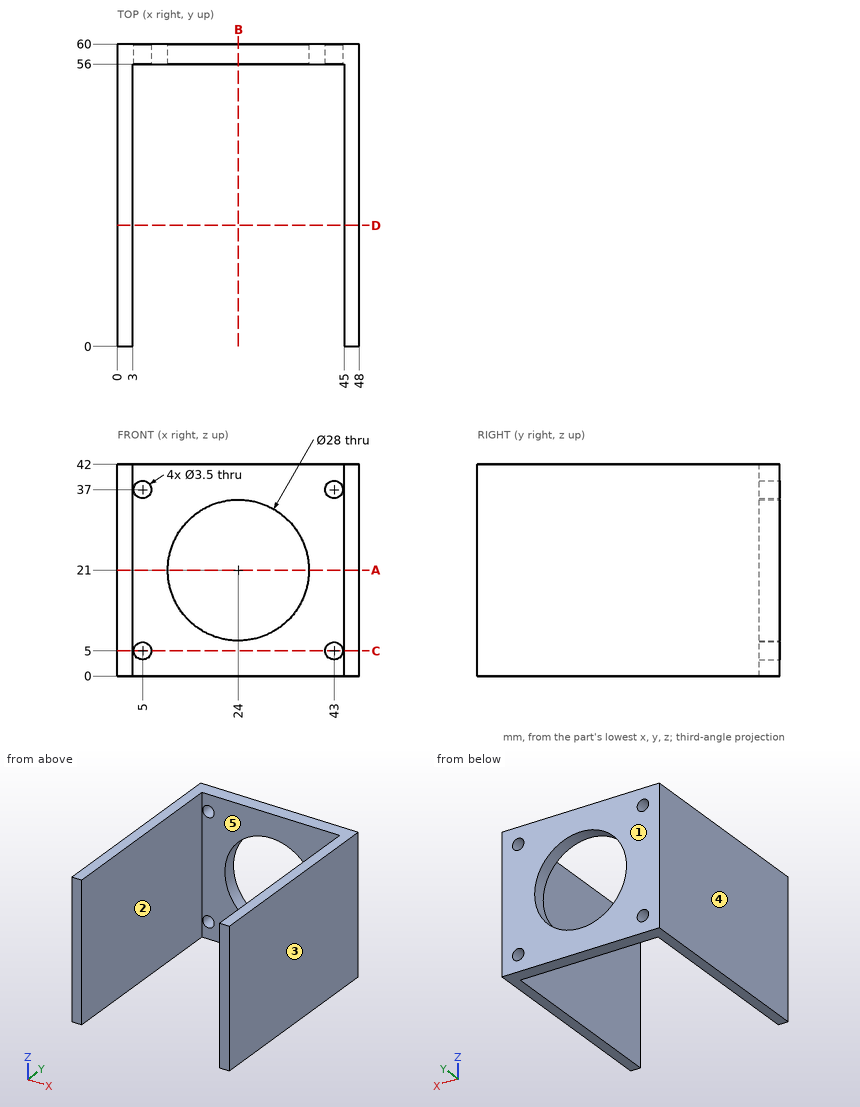
Source: three-view drawing plus pictorial views. Frame: mm from the lowest corner of the part. A direction names the side the tool comes from. Give positions to 0.01 mm unless a question says otherwise; leave off trailing zeros. Write each loop counter-clockwise with the first axis right and the second up, starting at its lowest first coordinate (ties: lowest second). Pieces come first, ordered by that corner, then holes. Notation, with made-up numbers: (40, -30.75) - (86, -30.75) arc R15 ccw to (86, -24.75) - close; hole circle Ø3 at (51, 86). An arc over 180 degrees is marked (long way). Write item = value, one per line. Start each with the question number.
Q1. Pin query (flat end, axial travel): pin 1 Ø6 at (x, z) = (15, 8.5) entering from -Y. Return the tip coordinate at first contact, or that it passes through.
Q2. Cut plane C-C, the plane z = 5. Return loops of the section in (x, y).
Q3. Draft query along X for the marked faces 3, 4 and 5. Return one class per face: +X half, -X half, draft (parallel to the pull), parting line (faces both ways), or undercut.
Q4. Cut plane D-D, the plane y = 24. Return loops of the section in (x, z), then the cut area to 3 significant figures.
Q5. Material intervals for probe 1 along Z at (x, y) = (5, 59); probe 2 along X at (y, z) = (57.3, 5); probe 3 along X at (y, z) = (4, 30.5), sorted ascending.
Q6. Reachability of the marked faces 1 and 2 from +Z, -Z, +X, -X, +Y, -Y: full face, straight path, thin tool, end or side. Return the list, or none.
Q7. Cut plane A-A, the plane z = 21. Return loops of the section in (x, y).
Q8. Cut plane B-B, the plane x = 24. Return loops of the section in (y, z), then the cut area to 3 significant figures.
Computed values:
q1.pin_1 = 56
q2.outline = (0, 0) - (3, 0) - (3, 56) - (3.25, 56) - (3.25, 60) - (0, 60) - close; (6.75, 56) - (41.25, 56) - (41.25, 60) - (6.75, 60) - close; (44.75, 56) - (45, 56) - (45, 0) - (48, 0) - (48, 60) - (44.75, 60) - close
q3.face_3 = +X half
q3.face_4 = -X half
q3.face_5 = undercut
q4.outline = (0, 0) - (3, 0) - (3, 42) - (0, 42) - close; (45, 0) - (48, 0) - (48, 42) - (45, 42) - close
q4.area = 252 mm²
q5.probe_1 = 0 to 3.25, 6.75 to 35.25, 38.75 to 42
q5.probe_2 = 0 to 3.25, 6.75 to 41.25, 44.75 to 48
q5.probe_3 = 0 to 3, 45 to 48
q6.face_1 = +Z, -Z, +X, -X, +Y
q6.face_2 = +Z, -Z, -Y
q7.outline = (0, 0) - (3, 0) - (3, 56) - (10, 56) - (10, 60) - (0, 60) - close; (38, 56) - (45, 56) - (45, 0) - (48, 0) - (48, 60) - (38, 60) - close
q8.outline = (56, 0) - (60, 0) - (60, 7) - (56, 7) - close; (56, 35) - (60, 35) - (60, 42) - (56, 42) - close
q8.area = 56.0 mm²
